from build123d import *

# Parameters (mm, degrees)
EXTRUDE_1_DEPTH     = 2.6
SKETCH_3_W          = 2.3134287
SKETCH_3_H          = 1.168890291
EXTRUDE_2_DEPTH     = 1.6
EXTRUDE_START       = 6.8
EXTRUDE_3_DEPTH     = 6.8
SKETCH_5_W          = 10.486803681
SKETCH_5_H          = 4.741640899
CUT_EXTRUDE_1_DEPTH = 4
SKETCH_6_R          = 0.35
EXTRUDE_4_DEPTH     = 4.5
SKETCH_7_W          = 31.6
SKETCH_7_H          = 2
EXTRUDE_5_DEPTH     = 5.8
SKETCH_8_R          = 0.35
EXTRUDE_6_DEPTH     = 4.3
SKETCH_9_R          = 0.5
CUT_EXTRUDE_2_DEPTH = 14.3
SKETCH_10_R         = 0.35
EXTRUDE_7_DEPTH     = 2
CUT_EXTRUDE_3_DEPTH = 4


with BuildPart() as part:
    # 草图1 → 旋转1 (revolve)
    with BuildSketch(Plane.XY, mode=Mode.PRIVATE) as revolve_1_sk:
        Polygon((4, 0), (4, -6.75), (7.15, -6.75), (7.15, -6.025), (4.8, -6.025), (4.8, -0.725), (7.15, -0.725), (7.15, 0), align=None)
    revolve(revolve_1_sk.sketch.rotate(Axis((0, 5.836385512, 0), (0, -1, 0)), 90), axis=Axis((0, 5.836385512, 0), (0, -1, 0)))

    # 草图2 → 凸台-拉伸1 (add)
    with BuildSketch(Plane(origin=(0, -0.725, 0), x_dir=(1, 0, 0), z_dir=(0, 1, 0))):
        with BuildLine():
            Line((5.314505692, -8.038664756), (7.251946558, -8.038664756))
            Line((7.251946558, -8.038664756), (7.251946558, -6.627550318))
            Line((7.251946558, -6.627550318), (6.099354415, -6.627550318))
            Line((6.099354415, -6.627550318), (6.099354415, -5.5))
            Line((6.099354415, -5.5), (2.051946558, -5.5))
            Line((2.051946558, -5.5), (2.051946558, -7.649656343))
            ThreePointArc((2.051946558, -7.649656343), (3.710373018, -7.616483358), (5.314505692, -8.038664756))
        make_face()
        with BuildLine():
            Line((-6.748053442, -5.5), (0.251946558, -5.5))
            Line((0.251946558, -5.5), (0.251946558, -8.240596845))
            ThreePointArc((0.251946558, -8.240596845), (-0.452097429, -8.666836759), (-1.091188438, -9.185412772))
            ThreePointArc((-1.091188438, -9.185412772), (-4.172119956, -8.255659578), (-6.748053442, -6.32663218))
            Line((-6.748053442, -6.32663218), (-6.748053442, -5.5))
        make_face()
    extrude(amount=EXTRUDE_1_DEPTH)

    # 草图3 → 凸台-拉伸2 (add)
    with BuildSketch(Plane(origin=(0, -0.725, 0), x_dir=(1, 0, 0), z_dir=(0, 1, 0))):
        with Locations((2.711416285, 6.407720863)):
            Rectangle(SKETCH_3_W, SKETCH_3_H)
    extrude(amount=EXTRUDE_2_DEPTH)

    # 草图4 → 凸台-拉伸3 (add)
    with BuildSketch(Plane.XZ.offset(6.025).offset(EXTRUDE_START)):
        with BuildLine():
            Line((-6.748053442, 6.32663218), (-6.748053442, 5.5))
            Line((-6.748053442, 5.5), (6.099354415, 5.5))
            Line((6.099354415, 5.5), (6.099354415, 6.627550318))
            Line((6.099354415, 6.627550318), (7.251946558, 6.627550318))
            Line((7.251946558, 6.627550318), (7.251946558, 8.038664756))
            Line((7.251946558, 8.038664756), (5.314505692, 8.038664756))
            ThreePointArc((5.314505692, 8.038664756), (1.942688245, 7.668176144), (-1.091188438, 9.185412772))
            ThreePointArc((-1.091188438, 9.185412772), (-4.172119956, 8.255659578), (-6.748053442, 6.32663218))
        make_face()
    extrude(amount=-EXTRUDE_3_DEPTH)

    # 草图5 → 切除-拉伸1 (cut)
    with BuildSketch(Plane.XZ.offset(12.825)):
        with Locations((0.182685526, 7.497044948)):
            Rectangle(SKETCH_5_W, SKETCH_5_H)
    extrude(amount=-CUT_EXTRUDE_1_DEPTH, mode=Mode.SUBTRACT)

    # 草图6 → 凸台-拉伸4 (add)
    with BuildSketch(Plane.XZ.offset(8.825)):
        with Locations(Location((3.019135042, 6.638228249, 0), (0, 0, 270))):
            Circle(SKETCH_6_R)
        with Locations(Location((0.019135042, 6.638228249, 0), (0, 0, 270))):
            Circle(SKETCH_6_R)
        with Locations(Location((-2.66722627, 7.973691801, 0), (0, 0, 270))):
            Circle(SKETCH_6_R)
    extrude(amount=EXTRUDE_4_DEPTH)

    # 草图7 → 凸台-拉伸5 (add)
    with BuildSketch(Plane(origin=(0, -6.025, 0), x_dir=(1, 0, 0), z_dir=(0, 1, 0))):
        with Locations((-2.8, 7.461335244)):
            Rectangle(SKETCH_7_W, SKETCH_7_H)
    extrude(amount=-EXTRUDE_5_DEPTH)

    # 草图8 → 凸台-拉伸6 (add)
    with BuildSketch(Plane.XZ.offset(11.825)):
        with Locations(Location((10.6, -7.444051339, 0), (0, 0, 270))):
            Circle(SKETCH_8_R)
        with Locations(Location((7.9, -7.444051339, 0), (0, 0, 270))):
            Circle(SKETCH_8_R)
        with Locations(Location((5.2, -7.444051339, 0), (0, 0, 270))):
            Circle(SKETCH_8_R)
    extrude(amount=EXTRUDE_6_DEPTH)

    # 草图9 → 切除-拉伸2 (cut)
    with BuildSketch(Plane.XZ.offset(11.825)):
        with Locations(Location((-15.3, -7.538758776, 0), (0, 0, 270))):
            Circle(SKETCH_9_R)
        with Locations(Location((-12.5, -7.538758776, 0), (0, 0, 270))):
            Circle(SKETCH_9_R)
    extrude(amount=-CUT_EXTRUDE_2_DEPTH, mode=Mode.SUBTRACT)

    # 草图10 → 凸台-拉伸7 (add)
    with BuildSketch(Plane(origin=(0, 1.875, 0), x_dir=(1, 0, 0), z_dir=(0, 1, 0))):
        with Locations(Location((-4.248213346, -6.799713472, 0), (0, 0, 270))):
            Circle(SKETCH_10_R)
        with Locations(Location((-1.693600984, -7.663244411, 0), (0, 0, 270))):
            Circle(SKETCH_10_R)
    extrude(amount=EXTRUDE_7_DEPTH)

    # 草图11 → 切除-拉伸3 (cut)
    with BuildSketch(Plane(origin=(0, -6.025, 0), x_dir=(1, 0, 0), z_dir=(0, 1, 0))):
        with BuildLine():
            Line((-14.790486895, 7.538758776), (-14.790486895, 5.844589861))
            ThreePointArc((-14.790486895, 5.844589861), (-15.3, 5.335076756), (-15.809513105, 5.844589861))
            Line((-15.809513105, 5.844589861), (-15.809513105, 7.538758776))
            ThreePointArc((-15.809513105, 7.538758776), (-15.3, 8.048271881), (-14.790486895, 7.538758776))
        make_face()
        with BuildLine():
            Line((-12.019991798, 7.538758776), (-12.019991798, 5.628707126))
            ThreePointArc((-12.019991798, 5.628707126), (-12.5, 5.148698925), (-12.980008202, 5.628707126))
            Line((-12.980008202, 5.628707126), (-12.980008202, 7.538758776))
            ThreePointArc((-12.980008202, 7.538758776), (-12.5, 8.018766978), (-12.019991798, 7.538758776))
        make_face()
    extrude(amount=-CUT_EXTRUDE_3_DEPTH, mode=Mode.SUBTRACT)


solid = part.part
Part model, mm, in its own coordinate system. A direction names the side the tool comes from. Give positions to 0.01 mm unless a question says otherwise; leave off trailing zeros. Loops run counter-clockwise (first coordinate to the right, second up) from the corner with the lowest first, then second, coordinate; pieces in that order, holes last. Notation, with made-up numbers: (36, 13.5) -> (56, 13.5) arc R19 cw to (56, 24.5) -> close; hole circle Ø10 at (8.5, 79.25). An arc over 180 degrees is marked (long way). Write each question's results on one line, items separated by ' | '. Start each with the question number.
Q1. Band-saw the part on A-A on x = -12.5. List the corners of the cut face in (y, z) (3 decimals), plus the area to 3 significant figures.
Q2. Band-saw the part on B-B on x = 7.9. List the corners of the cut face in (y, z) (3 decimals), plus the area to 3 significant figures.
Q3. Which spindle directions (+Z, -Z, +X, -X, +Y, -Y) get a long thin tool onto all of the face, cutting with end or side? Do faces 4 (the face through (2.7, 0.4, -5.823)), 5 (the face through (-12.02, -8, -7)), 6 (the face through (6, -12.825, 7)), 7 (the face through (3.868, 0.1, -6.4)), 8 (the face through (3, 0.875, -6)). Say none if no direction does.
Q4. Wall check: L1, parallel to Y at x = 3, z = -4 (3 decimals); L2, parallel to Y at x = 3, z = 6.75 (3 decimals); L3, parallel to X at y = -9.5, z = 6.5. Give the ranges that are in metal, low to high.
Q5. Band-saw the part on C-C on x = -8. List the corners of the cut face in (y, z) (3 decimals), plus the area to 3 significant figures.
Q6. Pin check, flat tips, straight feed: P1, Ø2, axis at y = -3.5, z = 6, coming from the +X side; P2, Ø4, axis at x = -7.5, z = -4, coming from the -Y side; P3, Ø0.6, axis at x = 0, z = 6.5, coming from the -Y side (3 decimals); P4, Ø1.3, axis at y = 0, z = -6.5, coming from the +X side. Stop position of each tip, or through.
Q7. Pull direction X, two halves, no side cores. Call faces 1 (the face through (-5.061, -11, 7)), 2 (the face through (-4.05, -3.34, 2.58)), 3 (the face through (5, 1.875, 7)): +X half, -X half, draft (parallel to the pull), parting line (faces both ways), or undercut.
Results are:
1) outline: (-11.825, -8.461) -> (-6.025, -8.461) -> (-6.025, -8.039) -> (-11.825, -8.039) -> close; (-11.825, -7.039) -> (-10.025, -7.039) -> (-10.025, -6.461) -> (-11.825, -6.461) -> close | area: 3.49 mm²
2) outline: (-16.125, -7.794) -> (-11.825, -7.794) -> (-11.825, -8.461) -> (-6.025, -8.461) -> (-6.025, -6.461) -> (-11.825, -6.461) -> (-11.825, -7.094) -> (-16.125, -7.094) -> close | area: 14.6 mm²
3) face 4: +X, -X, +Y | face 5: +Z, +Y | face 6: +Z, +X, -Y | face 7: -Z, +X, +Y | face 8: -Z, +X, -X, +Y
4) L1: y = -6.75 to -6.025, -0.725 to 0 | L2: y = -13.325 to -6.025, -0.725 to 1.875 | L3: x = -6.58 to -5.06, -0.3 to 0.34, 2.7 to 3.34, 5.43 to 6.1
5) outline: (-11.825, -8.461) -> (-6.025, -8.461) -> (-6.025, -6.461) -> (-11.825, -6.461) -> close | area: 11.6 mm²
6) P1: passes through | P2: stops at y = -6.75 | P3: stops at y = -13.325 | P4: stops at x = 4.11
7) face 1: undercut | face 2: parting line | face 3: draft
